Design review of the part shown in the three views and the two pictorial views. Dimensions are in mm from the part's minimum x, y and z. A direction names the side the tool comes from. Give positions to 0.01 mm unless a question says otherwise; leave off trailing zeros. Order: outer loops, then holes, each group sorted by start corner. A loop starts at its lowest first (then second) coordinate and runs counter-clockwise, first axis right, second up.
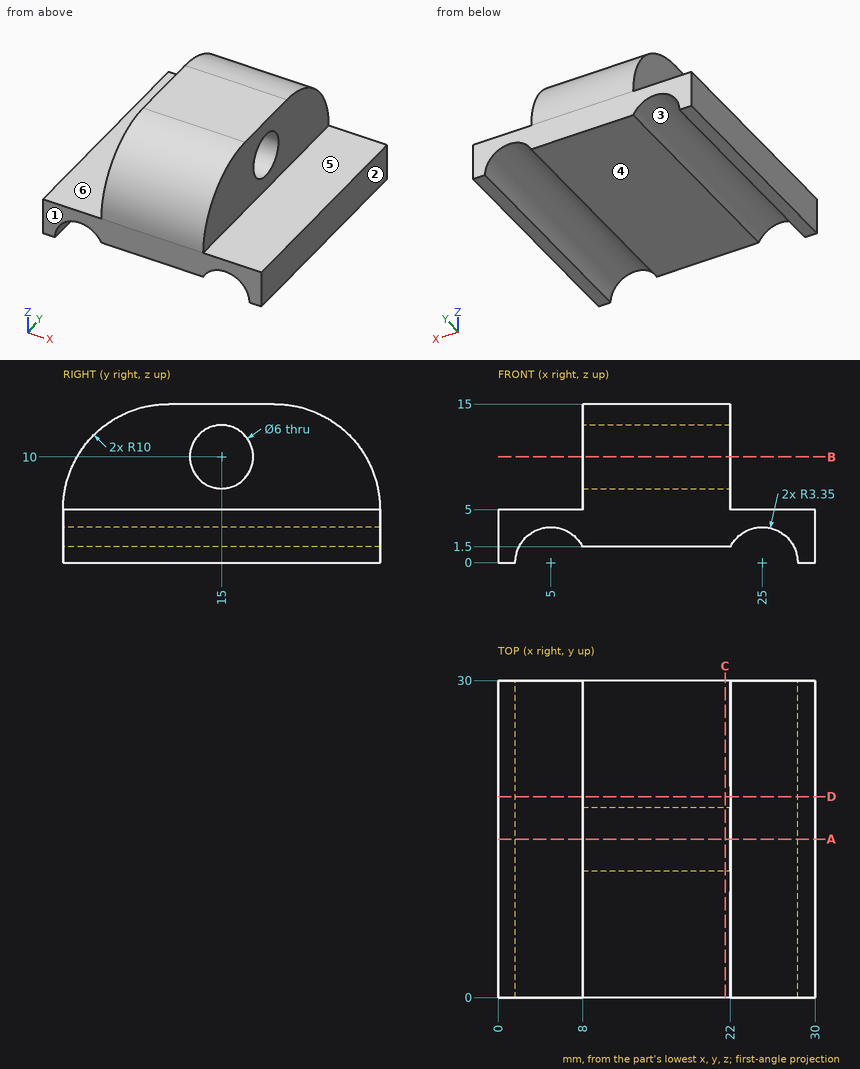
Item 1: Take a section at C-C (x = 21.5). Give the boundary of the cut face in (y, z).
Values found:
outline: (0, 1.5) - (30, 1.5) - (30, 5) arc R10 ccw to (20, 15) - (10, 15) arc R10 ccw to (0, 5) - close; hole circle Ø6 at (15, 10)
Item 2: For the marked faces 4, 5 and 6, list the 3-axis set-ups (+Z, -Z, +X, -X, +Y, -Y) from which the entire face can be reached by the end or side of a thin tool; tool diameter is ignored.
Values found:
face 4: -Z, +Y, -Y
face 5: +Z, +X, +Y, -Y
face 6: +Z, -X, +Y, -Y
Item 3: For line 1 (X direction, y = 21.75, z = 2.5); line 2 (X direction, y = 22, z = 2.25); line 3 (X direction, y = 5.5, z = 10.75), list the stretches that pass through material, from the lowest coordinate up.
Values found:
line 1: x = 0 to 2.77, 7.23 to 22.77, 27.23 to 30
line 2: x = 0 to 2.52, 7.48 to 22.52, 27.48 to 30
line 3: x = 8 to 22
Item 4: Take a section at D-D (y = 19). Give the boundary of the cut face in (x, z).
Values found:
outline: (0, 0) - (1.65, 0) arc R3.35 cw to (8, 1.5) - (22, 1.5) arc R3.35 cw to (28.35, 0) - (30, 0) - (30, 5) - (22, 5) - (22, 15) - (8, 15) - (8, 5) - (0, 5) - close
Item 5: Take a section at B-B (z = 10). Give the boundary of the cut face in (x, y), and give its area (3 significant figures).
Values found:
outline: (8, 1.34) - (22, 1.34) - (22, 12) - (8, 12) - close; (8, 18) - (22, 18) - (22, 28.66) - (8, 28.66) - close
area: 298 mm2
Item 6: Draft analysis for pull direction X (two halves, no side actions). For the marked faces 1, 2 and 3, state which applies: released by +X, released by -X, zero draft, split by the parting line, or undercut.
Values found:
face 1: zero draft
face 2: released by +X
face 3: undercut
Item 7: Clearance check with flat-ended pins moving along their axes: pin 1 Ø1.5 at (x, y) = (7.5, 24) entering from +Z; pin 2 Ø4 at (x, y) = (27, 11) entering from +Z; pin 3 Ø6 at (y, z) = (11, 12.5) entering from -X. State where each tip first meets the part, or that it passes through.
Values found:
pin 1: stops at z = 14.39
pin 2: stops at z = 5
pin 3: stops at x = 8
Item 8: Take a section at A-A (y = 15). Give the boundary of the cut face in (x, z), and give its area (3 significant figures).
Values found:
outline: (0, 0) - (1.65, 0) arc R3.35 cw to (8, 1.5) - (22, 1.5) arc R3.35 cw to (28.35, 0) - (30, 0) - (30, 5) - (22, 5) - (22, 7) - (8, 7) - (8, 5) - (0, 5) - close; (8, 13) - (22, 13) - (22, 15) - (8, 15) - close
area: 150 mm2
